from build123d import *

# Parameters (mm, degrees)
F0_R     = 14.2875
F1_DEPTH = 19.05
F2_R     = 15.875
F3_DEPTH = 2.54
F6_R     = 1.5875


with BuildPart() as f1:
    # F0 (on Top) → F1 (new body)
    with BuildSketch(Plane.XY):
        Circle(F0_R)
    extrude(amount=F1_DEPTH)

    # F2 (on face) → F3 (join)
    with BuildSketch(Plane(origin=(0, 0, 0), x_dir=(1, 0, 0), z_dir=(0, 0, -1))):
        Circle(F2_R)
    extrude(amount=-F3_DEPTH)

    # F4 (on Front) → F5 (revolve, cut)
    with BuildSketch(Plane.XZ):
        Polygon((0, 19.05), (0, 0), (5.08, 0), (5.08, 9.525), (7.9375, 19.05), align=None)
    revolve(axis=Axis((0, 0, 9.525), (0, 0, 1)), mode=Mode.SUBTRACT)

    # F6
    f6_edges = [f1.edges().sort_by_distance(p)[0] for p in [
        (-14.2875, 0, 19.05),
        (-7.9375, 0, 19.05),
        (-5.08, 0, 0),
    ]]
    fillet(f6_edges, radius=F6_R)


solid = f1.part
Geometry: final body of the model. Coordinates: model frame, mm. A direction names the side the tool comes from. Round coordinates to 2 decimals unless told otherwise and drop trailing zeros. Loops run counter-clockwise (first coordinate to the right, second up) from the corner with the lowest first, then second, coordinate; pieces in that order, holes last. Notation, with made-up numbers: (18, 54) -> (28, 54) arc R11 ccw to (28, 62) -> close; hole circle Ø2 at (48, 32). An arc over 180 degrees is marked (long way). One line per question, with ' | ' between items. Start each with the question number.
1. Set-up query: faces 5 (the face through (7, 0, 0)), 6 (the face through (-11.83, -8.31, 2.54)). Return all of +Z, -Z, +X, -X, +Y, -Y with unobstructed straight access to the full face (end or side cutting, diameter ignored); none if empty.
2. Contact query for flat-ended pins moving along their axis: pin 1 (1.5 mm diameter, centred on x = 1.5, z = 12, fed in from -Y); pin 2 (3 mm diameter, centred on x = 3, z = 3.5, fed in from -Y); pin 3 (13 mm diameter, centred on x = 0, y = 0, fed in from -Z). Output: stop coordinate, or through.
3. Mould query, pull axis X, two halves, no side actions, for faces 1 (the face through (-3, 9, 19.05)), 2 (the face through (-1.26, -5.66, 11.92)), 3 (the face through (-0.661, 5.037, 5.612)), 4 (the face through (-3.441, 15.497, 1.252)). Classes: pulls with the +X half, pulls with the -X half, needs draft (parallel to the pull), parting line crosses it, or undercut.
4. Section D-D on z = 10.25. Output: boundary loops of the cut face in (x, y) (1 decimal), and give its area (3 significant figures).
5. Section C-C on z = 6.25. Output: boundary loops of the cut face in (x, y) (1 decimal), and give its area (3 significant figures).
6. Line query: line 1 along Y through (x, z) = (0, 7); line 2 along Z through (x, y) = (11.5, 10); line 3 along X through (y, z) = (-2.5, 9.25). Output: solid intervals per line, ascending. Write a range as [from, to].
Returned:
1) face 5: -Z, +X, -X, +Y, -Y | face 6: +Z
2) pin 1: stops at y = -14.27 | pin 2: stops at y = -15.77 | pin 3: stops at z = 0.01
3) face 1: needs draft | face 2: undercut | face 3: undercut | face 4: parting line crosses it
4) outline: circle Ø28.6 at (0, 0); hole circle Ø10.6 at (0, 0) | area: 553 mm2
5) outline: circle Ø28.6 at (0, 0); hole circle Ø10.2 at (0, 0) | area: 560 mm2
6) line 1: y = [-14.29, -5.08], [5.08, 14.29] | line 2: z = [0, 2.54] | line 3: x = [-14.07, -4.42], [4.42, 14.07]
